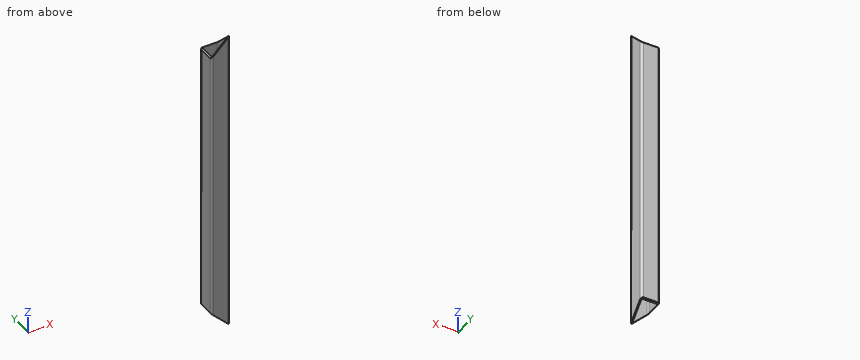
Autodesk Inventor part; units mm, degrees
ref_plane "Plano inicial" through (0, 0, -23.5401) normal (0, 0, 1) x (1, 0, 0)
ref_plane "Plano final" through (0, 0, 823.5401) normal (0, 0, 1) x (1, 0, 0)
ref_plane "Plano de trabajo4" through (25.4, 0, 825.4) normal (-0.7071, 0, 0.7071) x (0.7071, 0, 0.7071)
ref_plane "Plano inicial" through (0, 0, -23.5401) normal (0, 0, 1) x (1, 0, 0)
ref_plane "Plano final" through (0, 0, 823.5401) normal (0, 0, 1) x (1, 0, 0)
sketch "Boceto" plane through (0, 0, 0) normal (0, 0, 1) x (1, 0, 0)
  line L0 (-25.4, -19.05) -> (-25.4, 19.05)
  line L1 (-19.05, 25.4) -> (19.05, 25.4)
  line L2 (25.4, 19.05) -> (25.4, -19.05)
  line L3 (19.05, -25.4) -> (-19.05, -25.4)
  arc A0 (-25.4, -19.05) -> (-19.05, -25.4) centre (-19.05, -19.05) ccw
  arc A1 (-19.05, 25.4) -> (-25.4, 19.05) centre (-19.05, 19.05) ccw
  arc A2 (25.4, 19.05) -> (19.05, 25.4) centre (19.05, 19.05) ccw
  arc A3 (19.05, -25.4) -> (25.4, -19.05) centre (19.05, -19.05) ccw
  arc A4 (-19.05, 22.225) -> (-22.225, 19.05) centre (-19.05, 19.05) ccw
  line L4 (-19.05, 22.225) -> (19.05, 22.225)
  arc A5 (22.225, 19.05) -> (19.05, 22.225) centre (19.05, 19.05) ccw
  line L5 (22.225, 19.05) -> (22.225, -19.05)
  arc A6 (19.05, -22.225) -> (22.225, -19.05) centre (19.05, -19.05) ccw
  line L6 (19.05, -22.225) -> (-19.05, -22.225)
  arc A7 (-22.225, -19.05) -> (-19.05, -22.225) centre (-19.05, -19.05) ccw
  line L7 (-22.225, -19.05) -> (-22.225, 19.05)
  line L8 (0, 37.4012) -> (0, -37.4012) construction
  line L9 (-37.4012, 0) -> (37.4012, 0) construction
  dimension "d10" = 50.8
  dimension "d11" = 50.8
  dimension "d12" = 3.175
  dimension "d15" = 25.4
  dimension "d16" = 25.4
  dimension "d17" = 6.35
extrude "Cuerpo" add sketch "Boceto" along normal up to surface (847.0803 mm away) from surface at -23.5401
sketch "Sketch3" plane through (0, 0, 0) normal (0, 0, 1) x (1, 0, 0)
  line L0 (0, 0) -> (10, 0)
ref_plane "Work Plane3" through (0, 0, 0) normal (0, -1, 0) x (1, 0, 0)
ref_plane "Plano de trabajo4" through (25.4, 0, 825.4) normal (-0.7071, 0, 0.7071) x (0.7071, 0, 0.7071)
split "Dividir1" plane through (25.4, 0, 825.4) removes the side toward (-0.7071, 0, 0.7071)
ref_plane "Plano de trabajo5" through (25.4, 0, -25.4) normal (-0.7071, 0, -0.7071) x (-0.7071, 0, 0.7071)
split "Dividir2" plane through (25.4, 0, -25.4) removes the side toward (-0.7071, 0, -0.7071)
ref_plane "Plano de trabajo6" through (0, -25.4, 825.4) normal (0, 0.7071, 0.7071) x (1, 0, 0)
split "Dividir3" plane through (0, -25.4, 825.4) removes the side toward (0, 0.7071, 0.7071)
ref_plane "Plano de trabajo7" through (0, -25.4, -25.4) normal (0, 0.7071, -0.7071) x (1, 0, 0)
split "Dividir4" plane through (0, -25.4, -25.4) removes the side toward (0, 0.7071, -0.7071)
sketch "Sketch4" plane through (0, 0, 0) normal (0, -1, 0) x (1, 0, 0)
  line L0 (-2, -23.5401) -> (12, -23.5401)
  line L1 (-2, 823.5401) -> (12, 823.5401)
  dimension "d19" = 847.0803
equation "\"d10\" = G_H"
equation "\"d11\" = G_W"
equation "\"d12\" = G_T"
equation "\"d15\" = 0.5 * d10"
equation "\"d16\" = 0.5 * d11"
equation "\"d17\" = G_IR"
equation "\"d3\" = G_L"
equation "\"G_W\" = 50.8"
equation "\"G_H\" = 50.8"
equation "\"G_T\" = 3.175"
equation "\"G_IR\" = 6.35"
equation "\"G_L\" = d19"
equation "\"G_OFFSET_START\" = 23.54013"
equation "\"G_OFFSET_END\" = 23.54013"
equation "\"d13\" = -G_OFFSET_START"
equation "\"d14\" = G_OFFSET_END + B_L"
equation "\"B_L\" = 800"
properties part number "AISC - 2 x 2 x 1/8 - 33,35" material "Acero, suave"
Input: part model. Units: mm. Frame: model coordinates. Coordinates: 2 decimals unless noted, no trailing zeros. Order: outer loops, then holes, each group sorted by start corner. A loop starts at its lowest first (then second) coordinate and runs counter-clockwise, first axis right, second up. Notation, with made-up numbers: (-33.5, 20.5) - (3.5, 20.5) arc R16 ccw to (3.5, 50.5) - close; hole circle Ø10 at (38.25, 16.5). An arc over 180 degrees is marked (long way). Put each result on its own line as item: value.
1. Contact query for a flat-ended pin moving along its axis: pin 1 Ø10 at (x, y) = (12.5, 12) entering from +Z. Output: stop coordinate, or through.
Report:
pin 1: passes through
2. Cut plane A-A on x = -2. Return the cut outline in (y, z) (3 decimals).
Report:
outline: (-25.4, 2) - (-22.225, 2) - (-22.225, 798) - (-25.4, 798) - close; (22.225, 22.225) - (25.4, 25.4) - (25.4, 774.6) - (22.225, 777.775) - close
3. Cut plane B-B on y = 1.5. Return the cut outline in (x, z) (3 decimals).
Report:
outline: (-25.4, 25.4) - (-22.225, 22.225) - (-22.225, 777.775) - (-25.4, 774.6) - close; (22.225, 1.5) - (25.4, 1.5) - (25.4, 798.5) - (22.225, 798.5) - close
4. Line query: line 1 along Y through (x, z) = (3.5, 612.5) (3 decimals); line 2 along X through (y, z) = (-8, 25) (3 decimals). Output: solid intervals per line, ascending.
Report:
line 1: y = -25.4 to -22.225, 22.225 to 25.4
line 2: x = -25 to -22.225, 22.225 to 25.4
5. Cut plane C-C on z = 92. Return the cut outline in (x, y) (3 decimals), then the cut area to 3 significant figures.
Report:
outline: (-25.4, -19.05) arc R6.35 ccw to (-19.05, -25.4) - (19.05, -25.4) arc R6.35 ccw to (25.4, -19.05) - (25.4, 19.05) arc R6.35 ccw to (19.05, 25.4) - (-19.05, 25.4) arc R6.35 ccw to (-25.4, 19.05) - close; hole (-22.225, -19.05) arc R3.175 ccw to (-19.05, -22.225) - (19.05, -22.225) arc R3.175 ccw to (22.225, -19.05) - (22.225, 19.05) arc R3.175 ccw to (19.05, 22.225) - (-19.05, 22.225) arc R3.175 ccw to (-22.225, 19.05) - close
area: 579 mm2
